Autodesk Inventor part; units mm, degrees
ref_plane "YZ Plane" through (0, 0, 0) normal (1, 0, 0) x (0, 1, 0)
ref_plane "XZ Plane" through (0, 0, 0) normal (0, 1, 0) x (-1, 0, 0)
ref_plane "XY Plane" through (0, 0, 0) normal (0, 0, 1) x (1, 0, 0)
sketch "Sketch1" plane through (0, 0, 0) normal (0, 0, 1) x (1, 0, 0)
  line L0 (0, 0) -> (0, 3)
  line L1 (0, 3) -> (16, 3)
  line L2 (0, 0) -> (19, 0)
  line L3 (19, 0) -> (19, 30)
  line L4 (16, 3) -> (16, 30)
  line L5 (16, 30) -> (19, 30)
  dimension "d0" = 3
  dimension "d1" = 16
  dimension "d2" = 19
  dimension "d3" = 30
extrude "Extrusion1" add sketch "Sketch1" along normal blind 48
fillet "Fillet1" radius 10 2 edges at (17.5, 30, 0) (17.5, 30, 48)
sketch "Sketch2" plane through (19, 0, 48) normal (1, 0, 0) x (0, 0, -1)
  circle A0 centre (11, 20) radius 8.35
  circle A1 centre (37, 20) radius 8.35
  line L0 (48, 20) -> (48, 0)
  line L1 (38, 30) -> (10, 30)
  line L2 (0, 0) -> (0, 20)
  dimension "d7" = 16.7
  dimension "d8" = 16.7
  dimension "d9" = 11
  dimension "d10" = 10
  dimension "d11" = 10
  dimension "d12" = 11
extrude "Extrusion2" cut sketch "Sketch2" against normal blind 48
sketch "Sketch3" plane through (0, 3, 0) normal (0, 1, 0) x (1, 0, 0)
  circle A0 centre (7, -33) radius 1.5
  circle A1 centre (7, -15) radius 1.5
  line L0 (0, 0) -> (16, 0)
  line L1 (16, -48) -> (0, -48)
  line L2 (0, 0) -> (0, -48)
  dimension "d15" = 3
  dimension "d16" = 3
  dimension "d17" = 15
  dimension "d18" = 15
  dimension "d19" = 7
  dimension "d20" = 7
extrude "Extrusion3" cut sketch "Sketch3" against normal blind 48
Work out the finished part from the listing and answer in its coordinate system (mm). A direction names the side the tool comes from. Coordinates: 2 decimals unless noted, no trailing zeros. Write each loop counter-clockwise with the first axis right and the second up, starting at its lowest first coordinate (ties: lowest second). Pieces come first, ordered by that corner, then holes. Notation, with made-up numbers: (7, -33) - (34, -33) arc R19 cw to (34, -22) - close; hole circle Ø11 at (67, -4). An arc over 180 degrees is marked (long way). One line per question, with ' | ' between items.
1) Consider probe 1 along Z at (x, y) = (7, 2); probe 2 along Y at (x, z) = (17.75, 11); probe 3 along Z at (x, y) = (16.5, 12.5). Determine where each line is inside the solid, lowest interval first. Write a range as [from, to].
Checks:
probe 1: [0, 13.5], [16.5, 31.5], [34.5, 48] | probe 2: [0, 11.65], [28.35, 30] | probe 3: [0, 7.33], [14.67, 33.33], [40.67, 48]
2) The mould has two halves that part along X. Classify faces 1 (the face through (9, 0, 24)), 2 (the face through (0, 1, 24)), 3 (the face through (5.8, 1.5, 33.9)), 4 (the face through (5.5, 1.52, 14.93)): +X half, -X half, draft (parallel to the pull), parting line (faces both ways), or undercut.
Checks:
face 1: draft | face 2: -X half | face 3: undercut | face 4: undercut
3) Find section A-A, the plane z = 11. Determine the outline of the cut face in (x, y).
Checks:
outline: (0, 0) - (19, 0) - (19, 11.65) - (16, 11.65) - (16, 3) - (0, 3) - close; (16, 28.35) - (19, 28.35) - (19, 30) - (16, 30) - close
4) Flat-ended cylindrical pins translate along their axes: P1, Ø10, axis at y = 24, z = 24, coming from the -X side; P2, Ø10, axis at x = 4, z = 21, coming from the +Y side; P3, Ø13.5, axis at y = 20, z = 11, coming from the -X side. Find the tip coordinate at first contact, or state that the pin passes through.
Checks:
P1: x = 16 | P2: y = 3 | P3: through
5) Find section D-D, the plane y = 14.25. Determine the outline of the cut face in (x, z), and give its area (3 significant figures).
Checks:
outline: (16, 0) - (19, 0) - (19, 4.95) - (16, 4.95) - close; (16, 17.05) - (19, 17.05) - (19, 30.95) - (16, 30.95) - close; (16, 43.05) - (19, 43.05) - (19, 48) - (16, 48) - close | area: 71.3 mm2
6) For faces 5 (the face through (16, 13, 24)), 6 (the face through (17.52, 26.99, 2.85)), determine the directions among +Z, -Z, +X, -X, +Y, -Y from which every point of the face is accessible in a straight line to the end or side of a thin tool.
Checks:
face 5: +Z, -Z, -X, +Y | face 6: -Z, +X, -X, +Y
7) Find section C-C, the plane x = 17. Determine the outline of the cut face in (y, z).
Checks:
outline: (0, 0) - (20, 0) arc R10 ccw to (30, 10) - (30, 38) arc R10 ccw to (20, 48) - (0, 48) - close; hole circle Ø16.7 at (20, 11); hole circle Ø16.7 at (20, 37)
8) Find section B-B, the plane x = 7. Determine the outline of the cut face in (y, z).
Checks:
outline: (0, 0) - (3, 0) - (3, 13.5) - (0, 13.5) - close; (0, 16.5) - (3, 16.5) - (3, 31.5) - (0, 31.5) - close; (0, 34.5) - (3, 34.5) - (3, 48) - (0, 48) - close
